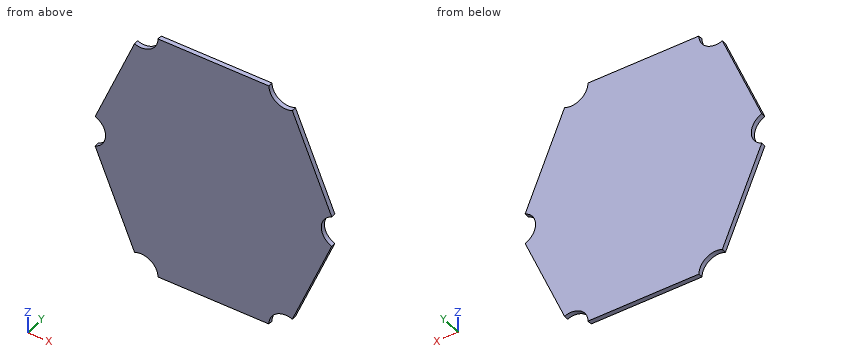
```python
from build123d import *

# Parameters (mm, degrees)
EXTRUDE_1_DEPTH     = 3
SKETCH_5_R          = 11
CUT_EXTRUDE_2_DEPTH = 116.299609713


with BuildPart() as part:
    # 草图4 → 凸台-拉伸1 (new body)
    with BuildSketch(Plane(origin=(0, 0, 0), x_dir=(1, 0, 0), z_dir=(0, 1, 0))):
        Polygon((-47, 82), (47, 82), (81, 0), (47, -82), (-47, -82), (-81, 0), align=None)
    extrude(amount=EXTRUDE_1_DEPTH)

    # 草图5 → 切除-拉伸2 (cut, through all)
    with BuildSketch(Plane(origin=(0, 3, 0), x_dir=(1, 0, 0), z_dir=(0, 1, 0))):
        with Locations((-81, 0)):
            Circle(SKETCH_5_R)
        with Locations((81, 0)):
            Circle(SKETCH_5_R)
        with Locations((47, -82)):
            Circle(SKETCH_5_R)
        with Locations((-47, -82)):
            Circle(SKETCH_5_R)
        with Locations((-47, 82)):
            Circle(SKETCH_5_R)
        with Locations((47, 82)):
            Circle(SKETCH_5_R)
    extrude(amount=-CUT_EXTRUDE_2_DEPTH, mode=Mode.SUBTRACT)


solid = part.part
```
The listing builds one solid part. Answer for the finished solid, in the listing's coordinates (mm). Give positions to 0.01 mm unless a question says otherwise; leave off trailing zeros. Write each loop counter-clockwise with the first axis right and the second up, starting at its lowest first coordinate (ties: lowest second). Pieces come first, ordered by that corner, then holes. Notation, with made-up numbers: (38.25, 27) - (51.25, 27) arc R34 ccw to (51.25, 60) - close; hole circle Ø1 at (-7.75, 70). An arc over 180 degrees is marked (long way). Use one line per item in the form item = value. Start each with the question number.
1) A flat-ended cylindrical pin translates along its axis: pin 1 Ø1.5 at (y, z) = (1.5, 34.5) entering from -X. Find the tip coordinate at first contact, or state that the pin passes through.
2) Find section C-C on z = -46.5. Determine the outline of the cut face in (x, y).
3) Find section B-B on x = -47. Determine the outline of the cut face in (y, z), plus the area to 3 significant figures.
4) Consider line 1 along X through (y, z) = (1.8, -26.5); line 2 along X through (y, z) = (0.7, 55.5); line 3 along Z through (x, y) = (-40, 0.35). Determine where each line is inside the solid, lowest interval first. Write a range as from..to.
5) Find section A-A on y = 1.35. Determine the outline of the cut face in (x, z).
Geometry results:
q1.pin_1 = -67.01
q2.outline = (-61.72, 0) - (61.72, 0) - (61.72, 3) - (-61.72, 3) - close
q3.outline = (0, -71) - (3, -71) - (3, 71) - (0, 71) - close
q3.area = 426 mm2
q4.line_1 = -70.01..70.01
q4.line_2 = -57.99..57.99
q4.line_3 = -73.51..73.51
q5.outline = (-76.79, -10.16) - (-51.21, -71.84) arc R11 cw to (-36, -82) - (36, -82) arc R11 cw to (51.21, -71.84) - (76.79, -10.16) arc R11 cw to (76.79, 10.16) - (51.21, 71.84) arc R11 cw to (36, 82) - (-36, 82) arc R11 cw to (-51.21, 71.84) - (-76.79, 10.16) arc R11 cw to start
